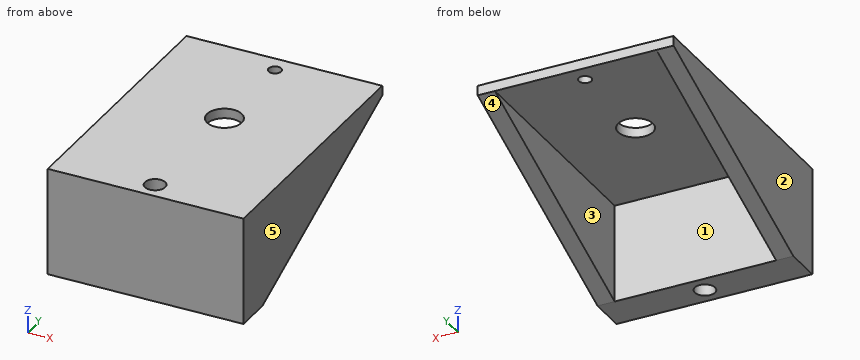
from build123d import *

# Parameters (mm, degrees)
SKETCH_1_W          = 80
SKETCH_1_H          = 110
EXTRUDE_1_DEPTH     = 4
SKETCH_2_R          = 7.1
SKETCH_2_R_2        = 2.6
CUT_EXTRUDE_1_DEPTH = 137.073509545
SKETCH_3_W          = 80
SKETCH_3_H          = 15
EXTRUDE_2_DEPTH     = 40
SKETCH_4_R          = 4.15
CUT_EXTRUDE_2_DEPTH = 143.954538228
EXTRUDE_3_DEPTH     = 7
EXTRUDE_4_DEPTH     = 7


with BuildPart() as part:
    # 草图1 → 凸台-拉伸1 (new body)
    with BuildSketch(Plane.XY):
        with Locations((40, -55)):
            Rectangle(SKETCH_1_W, SKETCH_1_H)
    extrude(amount=EXTRUDE_1_DEPTH)

    # 草图2 → 切除-拉伸1 (cut, through all)
    with BuildSketch(Plane.XY.offset(4)):
        with Locations((40, -47.5)):
            Circle(SKETCH_2_R)
        with Locations((40, -7.5)):
            Circle(SKETCH_2_R_2)
    extrude(amount=-CUT_EXTRUDE_1_DEPTH, mode=Mode.SUBTRACT)

    # 草图3 → 凸台-拉伸2 (add)
    with BuildSketch(Plane(origin=(0, 0, 0), x_dir=(-1, 0, 0), z_dir=(0, 0, -1))):
        with Locations((-40, -102.5)):
            Rectangle(SKETCH_3_W, SKETCH_3_H)
    extrude(amount=EXTRUDE_2_DEPTH)

    # 草图4 → 切除-拉伸2 (cut, through all)
    with BuildSketch(Plane(origin=(0, 0, -40), x_dir=(-1, 0, 0), z_dir=(0, 0, -1))):
        with Locations((-40, -102.5)):
            Circle(SKETCH_4_R)
    extrude(amount=-CUT_EXTRUDE_2_DEPTH, mode=Mode.SUBTRACT)

    # 草图5 → 凸台-拉伸3 (add)
    with BuildSketch(Plane(origin=(80, 0, 0), x_dir=(0, 0, -1), z_dir=(1, 0, 0))):
        Polygon((0, 0), (0, -95), (40, -95), align=None)
    extrude(amount=-EXTRUDE_3_DEPTH)

    # 草图6 → 凸台-拉伸4 (add)
    with BuildSketch(Plane.ZY):
        Polygon((0, 0), (0, -95), (-40, -95), align=None)
    extrude(amount=-EXTRUDE_4_DEPTH)


solid = part.part
Geometry check sheet. Reference: the model listing, model coordinates, mm. Face numbers are marked on the shaded views. A direction names the side the tool comes from. Round coordinates to 2 decimals unless told otherwise and drop trailing zeros. Order: outer loops, then holes, each group sorted by start corner. A loop starts at its lowest first (then second) coordinate and runs counter-clockwise, first axis right, second up. Notation, with made-up numbers: M -37.5,13.5 L -8.5,13.5 A20 cw -8.5,23.5 Z; hole C 12.25,67 d11. An arc over 180 degrees is marked long. Write each question's results on one line, items separated by ' | '. Start each with the question number.
1. Set-up check for the marked faces 1 and 2: record each of +Z, -Z, +X, -X, +Y, -Y from which the full face is reachable in a straight line by a thin tool's end or side.
2. Cross-section at A-A on x = 40. Record the boundary of the cut face in (y, z), plus the area to 3 significant figures.
3. Cross-section at D-D on x = 5. Record the boundary of the cut face in (y, z), plus the area to 3 significant figures.
4. Go/stop test with flat-tipped pins: P1, Ø11.5, axis at x = 40, y = -47.5, coming from the +Z side; P2, Ø20, axis at y = -62, z = -27.5, coming from the +X side; P3, Ø12, axis at x = 20.5, y = -27.5, coming from the -Z side. Record where each tip stops, or that it passes through.
5. Cross-section at B-B on y = -102.5. Record the boundary of the cut face in (x, z), plus the area to 3 significant figures.
6. Cross-section at C-C on z = -4. Record the boundary of the cut face in (x, y), plus the area to 3 significant figures.
7. Material ranges on L1, parallel to Y at x = 40, z = 1; L2, parallel to X at y = -40, z = -3.5; L3, parallel to Z at x = 54.5, y = -22.5, recorded low to high. Write a range as from..to.
8. Draft check along X on the marked faces 3, 4 and 5. Enter one of: pulls with the +X half, pulls with the -X half, needs draft (parallel to the pull), parting line crosses it, or undercut.
Resolved:
1) face 1: -Z, +Y | face 2: +Z, -Z, -X, +Y, -Y
2) outline: M -110,-40 L -106.65,-40 L -106.65,4 L -110,4 Z; M -98.35,-40 L -95,-40 L -95,0 L -54.6,0 L -54.6,4 L -98.35,4 Z; M -40.4,0 L -10.1,0 L -10.1,4 L -40.4,4 Z; M -4.9,0 L 0,0 L 0,4 L -4.9,4 Z | area: 597 mm2
3) outline: M -110,-40 L -95,-40 L 0,0 L 0,4 L -110,4 Z | area: 2,940 mm2
4) P1: through | P2: x = 80 | P3: z = 0
5) outline: M 0,-40 L 35.85,-40 L 35.85,4 L 0,4 Z; M 44.15,-40 L 80,-40 L 80,4 L 44.15,4 Z | area: 3,150 mm2
6) outline: M 0,-110 L 80,-110 L 80,-9.5 L 73,-9.5 L 73,-95 L 7,-95 L 7,-9.5 L 0,-9.5 Z; hole C 40,-102.5 d8.3 | area: 2,340 mm2
7) L1: -110..-106.65, -98.35..-54.6, -40.4..-10.1, -4.9..0 | L2: 0..7, 73..80 | L3: 0..4
8) face 3: undercut | face 4: needs draft | face 5: pulls with the +X half
